from build123d import *
from build123d.topology import SkipClean

# Parameters (mm, degrees)
SKETCH1_W                = 40
SKETCH1_H                = 27
BOSS_EXTRUDE1_DEPTH      = 30
CUT_EXTRUDE1_DEPTH       = 10
SKETCH3_R                = 2.5
CUT_EXTRUDE2_DEPTH       = 30
CUT_EXTRUDE5_START       = -10.62
CUT_EXTRUDE5_DEPTH       = 9
SKETCH10_W               = 20
SKETCH10_H               = 9
CUT_EXTRUDE7_DEPTH       = 6.8
SKETCH12_W               = 20
SKETCH12_H               = 9
CUT_EXTRUDE10_DEPTH      = 6.8
FILLET1_R                = 4
BOSS_EXTRUDE2_DEPTH      = 40
CUT_EXTRUDE14_DEPTH      = 54.078334793
CUT_EXTRUDE14_DEPTH_BACK = 54.078334793
SKETCH17_R               = 5.15
CUT_EXTRUDE11_REACH      = 42.583
SKETCH14_W               = 20
SKETCH14_H               = 10
SKETCH15_R               = 4.1
CUT_EXTRUDE12_DEPTH      = 4
SKETCH16_R               = 2.5
CUT_EXTRUDE13_DEPTH      = 4


with BuildPart() as part:
    # Sketch1 → Boss-Extrude1 (new body)
    with BuildSketch(Plane(origin=(0, 0, 0), x_dir=(1, 0, 0), z_dir=(0, 1, 0))):
        with Locations((-2.846153846, 4.313186813)):
            Rectangle(SKETCH1_W, SKETCH1_H)
    extrude(amount=BOSS_EXTRUDE1_DEPTH)

    # Sketch2 → Cut-Extrude1 (cut)
    with BuildSketch(Plane(origin=(0, 0, -17.813186813), x_dir=(-1, 0, 0), z_dir=(0, 0, -1))):
        Polygon((-8.086431081, 26), (-8.086431081, 4), (-0.206431081, 4), (-0.206431081, 7), (-2.866431081, 7), (-2.866431081, 8.008707537), (-0.253846154, 10.628707537), (5.946153846, 10.628707537), (8.558738773, 8.008707537), (8.558738773, 7), (5.898738773, 7), (5.898738773, 4), (13.778738773, 4), (13.778738773, 26), (5.898738773, 26), (5.898738773, 23), (8.558738773, 23), (8.558738773, 21.991292463), (5.938738773, 19.378707537), (-0.246431081, 19.378707537), (-2.866431081, 21.991292463), (-2.866431081, 23), (-0.206431081, 23), (-0.206431081, 26), align=None)
    extrude(amount=-CUT_EXTRUDE1_DEPTH, mode=Mode.SUBTRACT)

    # Sketch3 → Cut-Extrude2 (cut)
    with BuildSketch(Plane.XZ):
        with Locations(Location((10.423846154, 2.186813187, 0), (0, 0, 270))):
            Circle(SKETCH3_R)
        with Locations(Location((-16.116153846, 2.186813187, 0), (0, 0, 90))):
            Circle(SKETCH3_R)
    extrude(amount=-CUT_EXTRUDE2_DEPTH, mode=Mode.SUBTRACT)

    # Sketch8 → Cut-Extrude5 (cut)
    with BuildSketch(Plane.XZ.offset(CUT_EXTRUDE5_START)):
        with BuildLine():
            Line((3.282417725, 9.186813187), (17.153846154, 9.186813187))
            Line((17.153846154, 9.186813187), (17.153846154, -7.813186813))
            Line((17.153846154, -7.813186813), (10.423846154, -7.813186813))
            ThreePointArc((10.423846154, -7.813186813), (1.204301697, -1.686170159), (3.282417725, 9.186813187))
        make_face()
        with BuildLine():
            Line((-22.846153846, -7.813186813), (-16.116153846, -7.813186813))
            ThreePointArc((-16.116153846, -7.813186813), (-6.896609389, -1.686170159), (-8.974725418, 9.186813187))
            Line((-8.974725418, 9.186813187), (-22.846153846, 9.186813187))
            Line((-22.846153846, 9.186813187), (-22.846153846, -7.813186813))
        make_face()
    extrude(amount=-CUT_EXTRUDE5_DEPTH, mode=Mode.SUBTRACT)

    # Sketch10 → Cut-Extrude7 (cut)
    with BuildSketch(Plane.ZY.offset(-8.086431081)):
        with Locations((-7.813186813, 15.12)):
            Rectangle(SKETCH10_W, SKETCH10_H)
    extrude(amount=CUT_EXTRUDE7_DEPTH, mode=Mode.SUBTRACT)

    # Sketch12 → Cut-Extrude10 (cut)
    with BuildSketch(Plane(origin=(-13.778738773, 0, 0), x_dir=(0, 0, -1), z_dir=(1, 0, 0))):
        with Locations((7.813186813, 15.12)):
            Rectangle(SKETCH12_W, SKETCH12_H)
    extrude(amount=CUT_EXTRUDE10_DEPTH, mode=Mode.SUBTRACT)

    # Fillet1
    fillet1_edges = [part.edges().sort_by_distance(p)[0] for p in [
        (17.153846154, 24.81, 9.186813187),
        (-22.846153846, 24.81, 9.186813187),
        (17.153846154, 5.31, 9.186813187),
        (-22.846153846, 5.31, 9.186813187),
    ]]
    fillet(fillet1_edges, radius=FILLET1_R)

    # Sketch13 → Boss-Extrude2 (add)
    with BuildSketch(Plane(origin=(17.153846154, 0, 0), x_dir=(0, 0, -1), z_dir=(1, 0, 0))):
        with BuildLine():
            Line((17.813186813, -10), (17.813186813, 0))
            Line((17.813186813, 0), (15.195434711, 0))
            ThreePointArc((15.195434711, 0), (16.355078665, -1.690780832), (16.763186813, -3.7))
            ThreePointArc((16.763186813, -3.7), (9.603967646, -8.441891852), (8.030938916, 0))
            Line((8.030938916, 0), (2.813186813, 0))
            Line((2.813186813, 0), (2.813186813, -10))
            Line((2.813186813, -10), (17.813186813, -10))
        make_face()
    extrude(amount=-BOSS_EXTRUDE2_DEPTH)

    # Sketch17 → Cut-Extrude14 (cut, two sides: drawn at the far end of the back side and taken through both)
    with SkipClean():  # the faces are left unmerged after this step: merging them gives an invalid solid
        with BuildSketch(Plane(origin=(17.153846154, 0, 0), x_dir=(0, 0, -1), z_dir=(1, 0, 0)).offset(-CUT_EXTRUDE14_DEPTH_BACK)):
            with Locations((11.613186813, -3.7)):
                Circle(SKETCH17_R)
        extrude(amount=CUT_EXTRUDE14_DEPTH + CUT_EXTRUDE14_DEPTH_BACK, mode=Mode.SUBTRACT)

    # Sketch14 → Cut-Extrude11 (cut, up to next)
    with BuildSketch(Plane.XY.offset(-2.813186813), mode=Mode.PRIVATE) as cut_extrude11_sk1:
        with Locations((-2.846153846, -5)):
            Rectangle(SKETCH14_W, SKETCH14_H)
    cut_extrude11_tool1 = extrude(cut_extrude11_sk1.sketch, amount=-CUT_EXTRUDE11_REACH, mode=Mode.PRIVATE) & part.part
    add(cut_extrude11_tool1.solids().sort_by_distance((-2.846154, -5, -2.813187))[0], mode=Mode.SUBTRACT)

    # Sketch15 → Cut-Extrude12 (cut)
    with SkipClean():  # the faces are left unmerged after this step: merging them gives an invalid solid
        with BuildSketch(Plane(origin=(0, 30, 0), x_dir=(1, 0, 0), z_dir=(0, 1, 0))):
            with Locations(Location((-16.116153846, -2.186813187, 0), (0, 0, 270))):
                Circle(SKETCH15_R)
            with Locations(Location((10.423846154, -2.186813187, 0), (0, 0, 90))):
                Circle(SKETCH15_R)
        extrude(amount=-CUT_EXTRUDE12_DEPTH, mode=Mode.SUBTRACT)

    # Sketch16 → Cut-Extrude13 (cut)
    # profile 1 of 2: a face of its own
    with SkipClean():  # the faces are left unmerged after this step: merging them gives an invalid solid
        with BuildSketch(Plane.XZ):
            Polygon((-13.749017742, -1.913186813), (-11.381881639, 2.186813187), (-13.749017742, 6.286813187), (-18.48328995, 6.286813187), (-20.850426054, 2.186813187), (-18.48328995, -1.913186813), align=None)
            with Locations(Location((-16.116153846, 2.186813187, 0), (0, 0, 270))):
                Circle(SKETCH16_R, mode=Mode.SUBTRACT)
        # profile 2 of 2: a face of its own
        with BuildSketch(Plane.XZ):
            Polygon((12.790982258, -1.913186813), (15.158118361, 2.186813187), (12.790982258, 6.286813187), (8.05671005, 6.286813187), (5.689573946, 2.186813187), (8.05671005, -1.913186813), align=None)
            with Locations(Location((10.423846154, 2.186813187, 0), (0, 0, 270))):
                Circle(SKETCH16_R, mode=Mode.SUBTRACT)
        extrude(amount=-CUT_EXTRUDE13_DEPTH, mode=Mode.SUBTRACT)


solid = part.part
Can you work these out from the model? Positions are in its coordinate system, mm. A direction names the side the tool comes from. Round coordinates to 2 decimals unless told otherwise and drop trailing zeros. Loops run counter-clockwise (first coordinate to the right, second up) from the corner with the lowest first, then second, coordinate; pieces in that order, holes last. Notation, with made-up numbers: (81.25, 32) - (121.25, 32) arc R31 cw to (121.25, 65) - close; hole circle Ø3 at (65, 28.5). An arc over 180 degrees is marked (long way). Write item = value, one per line. Start each with the question number.
(1) If we section it at A-A (y = 6): Please give me the cut outline in (x, z).
(2) For P1, Ø4, axis at x = 10.42, z = 2.19, coming from the -Y side; P2, Ø1, axis at x = 5, z = 5.5, coming from the -Y side; P3, Ø1.8, axis at y = 14.5, z = -6, coming from the +X side; P4, Ø9, axis at x = -15, z = 0.5, coming from the -Y side, each with a flat end and sliding along its axis, tell me the tip position at first contact or that it passes through.
(3) If we section it at B-B (x = -17.5): Please give me the cut outline in (y, z), and give its area (3 significant figures).
(4) If we mould it in two halves opening along Z, with no side actions, what happens to faces 1 (the face through (-20.12, 28.03, 1.3)), 2 (the face through (-21.71, 5.38, 7.98)), 3 (the face through (-5.899, 6, -13))? For each: released by +Z, released by -Z, zero draft, split by the parting line, or undercut.
(5) For faces 4 (the face through (0.206, 24, -13)), 5 (the face through (10, 2, -1.913)), 6 (the face through (-16.23, 7.26, -0.31)), 7 (the face through (14.426, 28.028, 3.076)), 8 (the face through (16, 25, 8)), which set-ups out of +Z, -Z, +X, -X, +Y, -Y let a thin tool reach every point of the face, with its end or its side?
(6) If I drill on probe 1 along Y at (x, z) = (-15, -1); probe 2 along Z at (x, y) = (9, -4); probe 3 along Y at (x, z) = (4, 1.75), over which ranges is the centre line in solid material (lowest first)? Write a range as [from, to].
(7) If we section it at C-C (z = -3.75): Please give me the cut outline in (x, y), and give its area (3 significant figures).
(8) If we section it at D-D (z = -14.25): Give the number of separate pieces and of enclosed holes in the cut face, and give its area (3 significant figures).
Ans:
q1.outline = (-22.85, -17.81) - (-13.78, -17.81) - (-13.78, -7.81) - (-5.9, -7.81) - (-5.9, -17.81) - (0.21, -17.81) - (0.21, -7.81) - (8.09, -7.81) - (8.09, -17.81) - (17.15, -17.81) - (17.15, 5.19) arc R4 ccw to (13.15, 9.19) - (-18.85, 9.19) arc R4 ccw to (-22.85, 5.19) - close; hole circle Ø5 at (-16.12, 2.19); hole circle Ø5 at (10.42, 2.19)
q2.P1 = through
q2.P2 = 0
q2.P3 = 1.29
q2.P4 = -10
q3.outline = (-10, -17.81) - (30, -17.81) - (30, -1.67) - (26, -1.67) - (26, 0.1) - (19.62, 0.1) - (19.62, -7.81) - (10.62, -7.81) - (10.62, 0.1) - (4, 0.1) - (4, -1.91) - (0, -1.91) - (0, -2.81) - (-10, -2.81) - close; (0, 6.29) - (4, 6.29) - (4, 4.27) - (10.62, 4.27) - (10.62, 9.19) - (0, 9.19) - close; (19.62, 4.27) - (26, 4.27) - (26, 6.05) - (30, 6.05) - (30, 9.19) - (19.62, 9.19) - close; hole circle Ø10.3 at (-3.7, -11.61)
q3.area = 606 mm²
q4.face_1 = undercut
q4.face_2 = released by +Z
q4.face_3 = zero draft
q5.face_4 = -Z
q5.face_5 = -Y
q5.face_6 = +Y, -Y
q5.face_7 = +Y
q5.face_8 = +Z, +X, +Y, -Y
q6.probe_1 = [4, 10.62], [19.62, 26]
q6.probe_2 = [-17.81, -16.75], [-6.47, -2.81]
q6.probe_3 = [0, 10.62], [19.62, 30]
q7.outline = (-22.85, -10) - (-12.85, -10) - (-12.85, 0) - (7.15, 0) - (7.15, -10) - (17.15, -10) - (17.15, 10.62) - (1.29, 10.62) - (1.29, 19.62) - (17.15, 19.62) - (17.15, 30) - (-22.85, 30) - (-22.85, 19.62) - (-6.98, 19.62) - (-6.98, 10.62) - (-22.85, 10.62) - close
q7.area = 1,110 mm²
q8.separate_pieces = 3
q8.enclosed_holes = 1
q8.area = 833 mm²
